Design review of the part built by this model. Coordinates are the model's own, in mm. Coordinates: 2 decimals unless noted, no trailing zeros. Loops run counter-clockwise (first coordinate to the right, second up) from the corner with the lowest first, then second, coordinate; pieces in that order, holes last. Notation, with made-up numbers: (87, 3) -> (124, 3) arc R25 cw to (124, 26) -> close; hole circle Ø9 at (-11, 3.25). An arc over 180 degrees is marked (long way). Answer in a Markdown table with one row per item.
Autodesk Inventor part; units mm, degrees
ref_plane "YZ Plane" through (0, 0, 0) normal (1, 0, 0) x (0, 1, 0)
ref_plane "XZ Plane" through (0, 0, 0) normal (0, 1, 0) x (-1, 0, 0)
ref_plane "XY Plane" through (0, 0, 0) normal (0, 0, 1) x (1, 0, 0)
sketch "Sketch1" plane through (0, 0, 0) normal (0, 0, 1) x (1, 0, 0)
  line L0 (0, 0) -> (25.4, 0)
  line L1 (25.4, 0) -> (25.4, -24.13)
  line L2 (25.4, -24.13) -> (0, -24.13)
  line L3 (0, -24.13) -> (0, 0)
  dimension "d0" = 25.4
  dimension "d1" = 24.13
extrude "Extrusion1" add sketch "Sketch1" along normal blind 1.905
sketch "Sketch2" plane through (0, 0, 1.905) normal (0, 0, 1) x (1, 0, 0)
  circle A0 centre (1.905, -22.225) radius 0.9525
  circle A1 centre (1.905, -9.525) radius 0.9525
  circle A2 centre (23.495, -9.525) radius 0.9525
  circle A3 centre (23.495, -22.225) radius 0.9525
  line L0 (25.4, -24.13) -> (25.4, 0)
  line L1 (0, -24.13) -> (25.4, -24.13)
  line L2 (0, 0) -> (0, -24.13)
  line L3 (25.4, 0) -> (0, 0)
  dimension "d4" = 1.905
  dimension "d5" = 1.905
  dimension "d6" = 1.905
  dimension "d7" = 1.905
  dimension "d8" = 1.905
  dimension "d9" = 1.905
  dimension "d10" = 1.905
  dimension "d11" = 1.905
  dimension "d12" = 9.525
  dimension "d13" = 9.525
  dimension "d14" = 1.905
  dimension "d15" = 1.905
extrude "Extrusion2" cut sketch "Sketch2" against normal blind 1.905 contours A0 | A1 | A2 | A3
properties part number "CameraBoard" material "Thermoplastic Resin"
(1) Take a section at B-B on z = 0.4. Give the boundary of the cut face in (x, y) (1 decimal), and give its area (4 significant figures).
Evaluation:
| item | result |
|---|---|
| outline | (0, -24.1) -> (25.4, -24.1) -> (25.4, 0) -> (0, 0) -> close; hole circle Ø1.9 at (1.9, -22.2); hole circle Ø1.9 at (1.9, -9.5); hole circle Ø1.9 at (23.5, -22.2); hole circle Ø1.9 at (23.5, -9.5) |
| area | 601.5 mm² |
(2) To check wall thickness, follow probe 1 along X at (y, z) = (-9.25, 1.45). State the ranges of the line that lie inside material, in increasing order.
Evaluation:
| item | result |
|---|---|
| probe 1 | x = 0 to 0.99, 2.82 to 22.58, 24.41 to 25.4 |
(3) Take a section at A-A on x = 23.5. Give the boundary of the cut face in (y, z) (3 decimals).
Evaluation:
| item | result |
|---|---|
| outline | (-24.13, 0) -> (-23.177, 0) -> (-23.177, 1.905) -> (-24.13, 1.905) -> close; (-21.273, 0) -> (-10.477, 0) -> (-10.477, 1.905) -> (-21.273, 1.905) -> close; (-8.573, 0) -> (0, 0) -> (0, 1.905) -> (-8.573, 1.905) -> close |
(4) Draft analysis for pull direction Y (two halves, no side actions). For faces 1 (the flat face through (25.4, -12, 1)), 2 (the cylindrical face through (22.543, -9.483, 0.966)), 3 (the cylindrical face through (22.739, -22.805, 0.966)), 4 (the flat face through (13, -24.13, 1)), state which applies: pulls with the +Y half, pulls with the -Y half, needs draft (parallel to the pull), parting line crosses it, or undercut.
Evaluation:
| item | result |
|---|---|
| face 1 | needs draft |
| face 2 | undercut |
| face 3 | undercut |
| face 4 | pulls with the -Y half |
